Could you check a few things on this drawing? It's one solid part, dimensions in mm from its lowest x, y, z. A direction names the side the tool comes from. Give positions to 0.01 mm unless a question says otherwise; leave off trailing zeros. Write each loop counter-clockwise with the first axis right and the second up, starting at its lowest first coordinate (ties: lowest second). Pieces come first, ordered by that corner, then holes. Notation, with made-up numbers: M 21,-34 L 63,-34 A27 cw 63,-6 Z; hole C 29,70 d5. An arc over 180 degrees is marked long. Answer as CSV lines item,"result". Start each with the question number.
Q1. Suppose I cut it at B-B (z = 17). Write out the boundary of the cut face in (x, y) (1 decimal).
Q2. On a 3-axis mill with a long thin cutter (end or side, diameter ignored), from which of +Z, -Z, +X, -X, +Y, -Y can I reach the whole of each face in a straight line? I mean the marked faces 1 and 2. Say none if no direction works.
Q3. Suppose I cut it at C-C (x = 55). Write out the boundary of the cut face in (y, z), then the cut area to 3 significant figures.
Q4. Thinking about a two-plate mould opening in X: for the marked faces 3, 4, 5 and 6, which applies, +X half, -X half, draft (parallel to the pull), parting line (faces both ways), or undercut?
Q5. For pin 1 (20.5 mm diameter, centred on x = 49, z = 16, fed in from +Y); pin 2 (4 mm diameter, centred on x = 36, y = 53, fed in from +Z); pin 3 (10 mm diameter, centred on x = 93, y = 13, fed in from -Z), each with a flat end and sliding along its axis, tell me the tip position at first contact or that it passes through.
Q6. If I drill on line 1 along X through (y, z) = (70.5, 26) (1 decimal); line 2 along Y through (x, z) = (71, 27.5); line 3 along X through (y, z) = (77.5, 17) (1 decimal), over which ranges is the centre line in solid material (lowest first)?
Q7. Suppose I cut it at A-A (y = 46.5). Write out the boundary of the cut face in (x, z) (1 decimal), then the cut area to 3 significant figures.
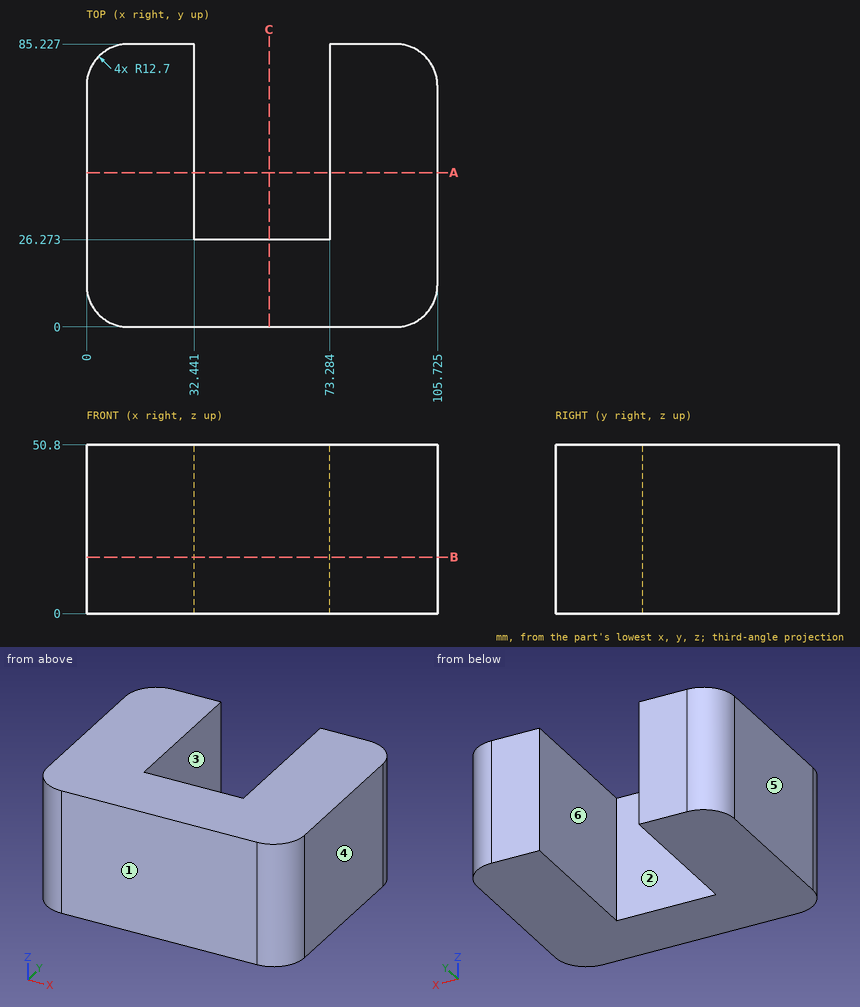
Resolved:
1,outline,"M 0,12.7 A12.7 ccw 12.7,0 L 93,0 A12.7 ccw 105.7,12.7 L 105.7,72.5 A12.7 ccw 93,85.2 L 73.3,85.2 L 73.3,26.3 L 32.4,26.3 L 32.4,85.2 L 12.7,85.2 A12.7 ccw 0,72.5 Z"
2,face 1,"+Z, -Z, +X, -X, -Y"
2,face 2,"+Z, -Z, +Y"
3,outline,"M 0,0 L 26.27,0 L 26.27,50.8 L 0,50.8 Z"
3,area,"1,330 mm^2"
4,face 3,"undercut"
4,face 4,"+X half"
4,face 5,"-X half"
4,face 6,"undercut"
5,pin 1,"y = 26.27"
5,pin 2,"through"
5,pin 3,"z = 0"
6,line 1,"0 to 32.4, 73.3 to 105.7"
6,line 2,"0 to 26.27"
6,line 3,"1 to 32.4, 73.3 to 104.7"
7,outline,"M 0,0 L 32.4,0 L 32.4,50.8 L 0,50.8 Z; M 73.3,0 L 105.7,0 L 105.7,50.8 L 73.3,50.8 Z"
7,area,"3,300 mm^2"
